Verification items for the finished model (mm, model axes). Face numbers are marked on the shaded views. A direction names the side the tool comes from. Coordinates: 2 decimals unless noted, no trailing zeros. Loops run counter-clockwise (first coordinate to the right, second up) from the corner with the lowest first, then second, coordinate; pieces in that order, holes last. Notation, with made-up numbers: (-13.75, -5) - (-1.75, -5) arc R5 cw to (-1.75, 0) - close; hole circle Ø2 at (48, -23). An arc over 180 degrees is marked (long way). Answer as CSV lines item,"result". Start each with the question number.
1. Material ranges on line 1 (Y direction, x = 2.75, z = 2.7) (1 decimal); line 2 (X direction, y = 2.5, z = 3.55); line 3 (Y direction, x = 3.5, z = 3.9) (1 decimal), recorded low to high. Write a range as [from, to].
2. Set-up check for the marked faces 4, 5 and 6: record each of +Z, -Z, +X, -X, +Y, -Y from which the full face is reachable in a straight line by a thin tool's end or side.
3. Cross-section at B-B (y = 2.5). Enter the section's corners in (x, z), plus the area to 3 significant figures.
4. Cross-section at A-A (x = 2.75). Enter the section's corners in (y, z) (1 decimal).
5. Cross-section at C-C (z = 2.9). State how many separate pieces and enclosed holes the cut face has, plus the area to 3 significant figures.
6. Cross-section at D-D (y = 8). Enter the section's corners in (x, z), plus the area to 3 significant figures.
7. Gauge pin test, flat ends, axial feed: P1, Ø0.6, axis at x = 1.5, z = 3.5, coming from the -Y side; P2, Ø1.4, axis at x = 13.45, y = 12.145, coming from the -Z side; P3, Ø1, axis at y = 7, z = 3.5, coming from the -X side; P4, Ø0.6, axis at y = 7, z = 3, coming from the +X side. Record the tip position at first contact, or that the pin passes through.
8. Release check for a two-part mould opening along Y. For the marked faces 1, 2 and 3 record: pulls with the +Y half, pulls with the -Y half, needs draft (parallel to the pull), parting line crosses it, or undercut.
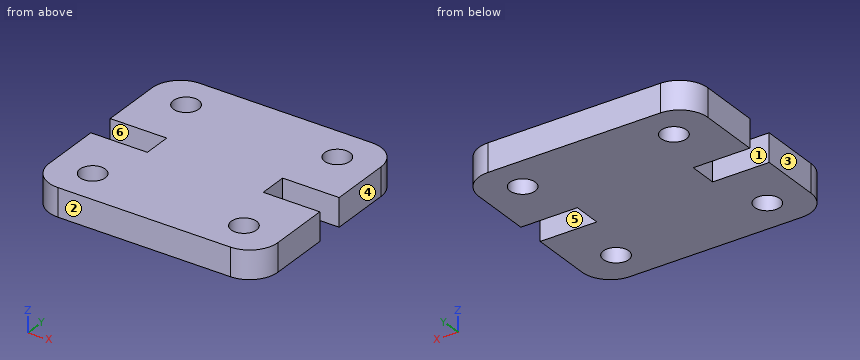
```python
from build123d import *

# Parameters (mm, degrees)
SKETCH1_R           = 0.9
BOSS_EXTRUDE1_DEPTH = 4
SKETCH2_W           = 16.2
SKETCH2_H           = 14.645
CUT_EXTRUDE1_DEPTH  = 2


with BuildPart() as part:
    # Sketch1 → Boss-Extrude1 (new body)
    with BuildSketch(Plane.XY):
        with BuildLine():
            Line((2, 14.645), (14.2, 14.645))
            ThreePointArc((14.2, 14.645), (15.614213562, 14.059213562), (16.2, 12.645))
            Line((16.2, 12.645), (16.2, 8.3225))
            Line((16.2, 8.3225), (12.2, 8.3225))
            Line((12.2, 8.3225), (12.2, 6.3225))
            Line((12.2, 6.3225), (16.2, 6.3225))
            Line((16.2, 6.3225), (16.2, 2))
            ThreePointArc((16.2, 2), (15.614213562, 0.585786438), (14.2, 0))
            Line((14.2, 0), (2, 0))
            ThreePointArc((2, 0), (0.585786438, 0.585786438), (0, 2))
            Line((0, 2), (0, 6.3225))
            Line((0, 6.3225), (4, 6.3225))
            Line((4, 6.3225), (4, 8.3225))
            Line((4, 8.3225), (0, 8.3225))
            Line((0, 8.3225), (0, 12.645))
            ThreePointArc((0, 12.645), (0.585786438, 14.059213562), (2, 14.645))
        make_face()
        with Locations((2.75, 12.145)):
            Circle(SKETCH1_R, mode=Mode.SUBTRACT)
        with Locations((13.45, 2.5)):
            Circle(SKETCH1_R, mode=Mode.SUBTRACT)
        with Locations((13.45, 12.145)):
            Circle(SKETCH1_R, mode=Mode.SUBTRACT)
        with Locations((2.75, 2.5)):
            Circle(SKETCH1_R, mode=Mode.SUBTRACT)
    extrude(amount=BOSS_EXTRUDE1_DEPTH)

    # Sketch2 → Cut-Extrude1 (cut)
    with BuildSketch(Plane(origin=(0, 0, 0), x_dir=(-1, 0, 0), z_dir=(0, 0, -1))):
        with Locations((-8.1, 7.3225)):
            Rectangle(SKETCH2_W, SKETCH2_H)
    extrude(amount=-CUT_EXTRUDE1_DEPTH, mode=Mode.SUBTRACT)


solid = part.part
```
Values follow:
1,line 1,"y = [0, 1.6], [3.4, 6.3], [8.3, 11.2], [13, 14.6]"
1,line 2,"x = [0, 1.85], [3.65, 12.55], [14.35, 16.2]"
1,line 3,"y = [0, 2], [3, 6.3], [8.3, 11.6], [12.6, 14.6]"
2,face 4,"+Z, -Z, +X, +Y, -Y"
2,face 5,"+Z, -Z, +X"
2,face 6,"+Z, -Z, -X"
3,outline,"(0, 2) - (1.85, 2) - (1.85, 4) - (0, 4) - close; (3.65, 2) - (12.55, 2) - (12.55, 4) - (3.65, 4) - close; (14.35, 2) - (16.2, 2) - (16.2, 4) - (14.35, 4) - close"
3,area,"25.2 mm²"
4,outline,"(0, 2) - (1.6, 2) - (1.6, 4) - (0, 4) - close; (3.4, 2) - (6.3, 2) - (6.3, 4) - (3.4, 4) - close; (8.3, 2) - (11.2, 2) - (11.2, 4) - (8.3, 4) - close; (13, 2) - (14.6, 2) - (14.6, 4) - (13, 4) - close"
5,separate pieces,"1"
5,enclosed holes,"4"
5,area,"208 mm²"
6,outline,"(4, 2) - (12.2, 2) - (12.2, 4) - (4, 4) - close"
6,area,"16.4 mm²"
7,P1,"stops at y = 0.01"
7,P2,"passes through"
7,P3,"stops at x = 4"
7,P4,"stops at x = 12.2"
8,face 1,"undercut"
8,face 2,"pulls with the -Y half"
8,face 3,"needs draft"
